Part print with two shaded views. Sizes in mm from the minimum x, y, z corner. Coordinates: 2 decimals unless noted, no trailing zeros. Write each loop counter-clockwise with the first axis right and the second up, starting at its lowest first coordinate (ties: lowest second). Pieces come first, ordered by that corner, then holes. Notation, with made-up numbers: M 45,-5 L 96,-5 A13 ccw 96,15 Z; hole C 89,-5 d7. An arc over 180 degrees is marked long. One line per question, with ' | ' between items. Start each with the question number.
(1) Flat gauge pin, fed straight in: pin 1 Ø1 at (x, z) = (238.5, 8) entering from -Y. Where does the tip first touch, or does it go through?
(2) Cut at B-B (x = 149). Write the cut outline in (y, z) (3 decimals), plus the area to 3 significant figures.
(3) Wall check: probe 1 along Y at (x, z) = (119, 15.25) (3 decimals); probe 2 along Z at (x, y) = (170, 46.5) (3 decimals). Give the ranges that are in metal, low to high.
(4) Cut at A-A (z = 16). Write the cut outline in (x, y) (3 decimals), plus the area to 3 significant figures.
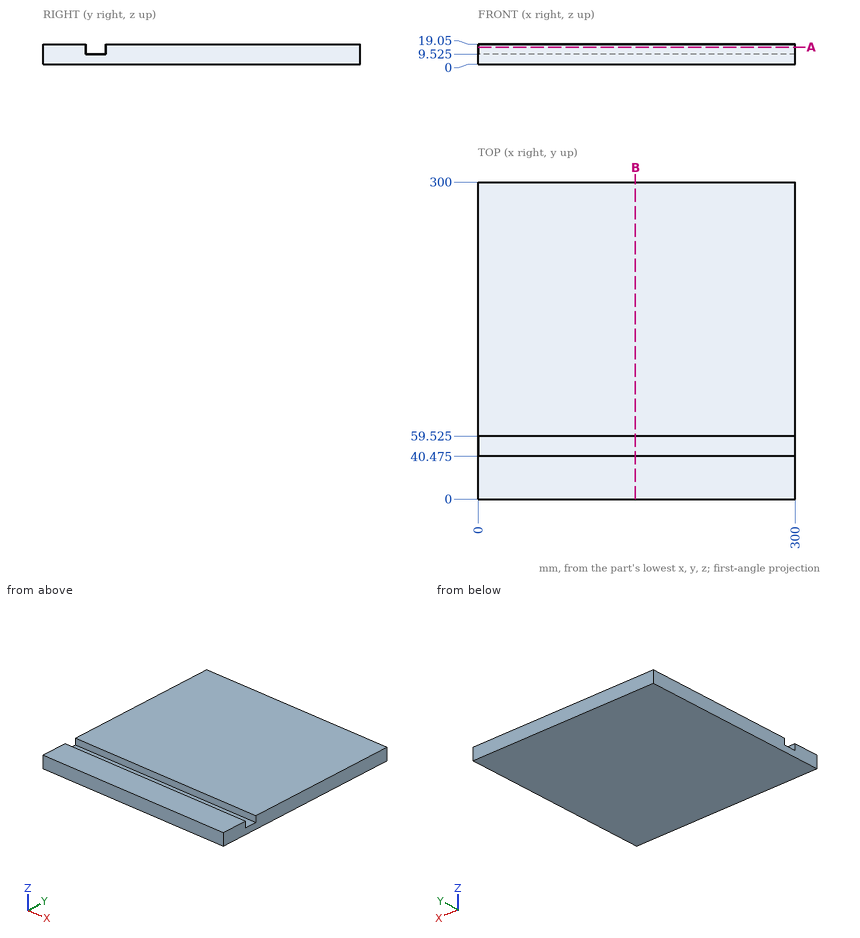
Filled in:
1) pin 1: y = 0
2) outline: M 0,0 L 300,0 L 300,19.05 L 59.525,19.05 L 59.525,9.525 L 40.475,9.525 L 40.475,19.05 L 0,19.05 Z | area: 5,530 mm²
3) probe 1: 0 to 40.475, 59.525 to 300 | probe 2: 0 to 9.525
4) outline: M 0,0 L 300,0 L 300,40.475 L 0,40.475 Z; M 0,59.525 L 300,59.525 L 300,300 L 0,300 Z | area: 84,300 mm²
